from build123d import *

# Parameters (mm, degrees)
F0_W      = 146.05
F0_H      = 127
F1_DEPTH  = 2.54
F2_W      = 146.05
F2_H      = 12.7
F3_DEPTH  = 50.8
F5_W      = 50.8
F5_H      = 28.575
F6_DEPTH  = 12.7
F7_W      = 50.8
F7_H      = 3.175
F7_H_2    = 12.7
F8_DEPTH  = 1.5875
F9_W      = 63.5
F9_H      = 50.8
F10_DEPTH = 2.54
F11_W     = 12.7
F11_H     = 73.025
F12_DEPTH = 50.8
F13_W     = 148.59
F13_H     = 2.54
F15_DEPTH = 57.15
F14_W     = 2.54
F14_H     = 127
F16_DEPTH = 57.15
F18_DEPTH = 50.8
F19_W     = 31.75
F19_H     = 12.7
F20_DEPTH = 50.8
F22_DEPTH = 50.8
F24_DEPTH = 50.8
F25_W     = 12.68959
F25_H     = 50.8
F26_DEPTH = 50.8
F4_W      = 15.875
F4_H      = 15.875
F27_DEPTH = 38.1
F28_W     = 85.09
F28_H     = 2.54
F29_DEPTH = 57.15
F30_W     = 2.54
F30_H     = 50.8
F32_DEPTH = 57.15
F31_W     = 63.5
F31_H     = 2.54
F33_DEPTH = 57.15
F34_W     = 2.54
F34_H     = 57.15
F35_DEPTH = 57.15


with BuildPart() as f1:
    # F0 (on Top) → F1 (new body)
    with BuildSketch(Plane.XY):
        Rectangle(F0_W, F0_H)
    extrude(amount=F1_DEPTH)

    # F2 (on face) → F3 (join)
    with BuildSketch(Plane.XY.offset(2.54)):
        with Locations((0, 57.15)):
            Rectangle(F2_W, F2_H)
    extrude(amount=F3_DEPTH)

    # F5 (on face) → F6 (cut)
    with BuildSketch(Plane.XZ.offset(-50.8)):
        with Locations((0, 35.8775)):
            Rectangle(F5_W, F5_H)
    extrude(amount=-F6_DEPTH, mode=Mode.SUBTRACT)

    # F7 (on face) → F8 (join)
    with BuildSketch(Plane.XY.offset(21.59)):
        with Locations((0, 49.2125)):
            Rectangle(F7_W, F7_H)
        with Locations((0, 57.15)):
            Rectangle(F7_W, F7_H_2)
    extrude(amount=F8_DEPTH)

    # F9 (on Top) → F10 (join)
    with BuildSketch(Plane.XY):
        with Locations((-41.275, -88.9)):
            Rectangle(F9_W, F9_H)
    extrude(amount=F10_DEPTH)

    # F11 (on face) → F12 (join)
    with BuildSketch(Plane.XY.offset(2.54)):
        with Locations((66.675, 14.2875)):
            Rectangle(F11_W, F11_H)
    extrude(amount=F12_DEPTH)

    # F13 (on Top) → F15 (join)
    with BuildSketch(Plane.XY):
        with Locations((1.27, 64.77)):
            Rectangle(F13_W, F13_H)
    extrude(amount=F15_DEPTH)

    # F14 (on Top) → F16 (join)
    with BuildSketch(Plane.XY):
        with Locations((74.295, 0)):
            Rectangle(F14_W, F14_H)
    extrude(amount=F16_DEPTH)

    # F17 (on face) → F18 (join)
    with BuildSketch(Plane.XY.offset(2.54)):
        Polygon((60.325, 31.75), (60.325, 50.8), (41.275, 50.8), align=None)
    extrude(amount=F18_DEPTH)

    # F19 (on face) → F20 (join)
    with BuildSketch(Plane.XY.offset(2.54)):
        with Locations((6.35, -57.15)):
            Rectangle(F19_W, F19_H)
    extrude(amount=F20_DEPTH)

    # F21 (on face) → F22 (join)
    with BuildSketch(Plane.XY.offset(2.54)):
        Polygon((34.925, -63.5), (22.225, -50.8), (22.225, -63.5), align=None)
    extrude(amount=F22_DEPTH)

    # F23 (on face) → F24 (join)
    with BuildSketch(Plane.XY.offset(2.54)):
        Polygon((-9.525, -63.5), (-9.525, -50.8), (-22.21459, -63.5), align=None)
    extrude(amount=F24_DEPTH)

    # F25 (on face) → F26 (join)
    with BuildSketch(Plane.XY.offset(2.54)):
        with Locations((-15.869795, -88.9)):
            Rectangle(F25_W, F25_H)
    extrude(amount=F26_DEPTH)

    # F4 (on face) → F27 (join)
    with BuildSketch(Plane.XY.offset(2.54)):
        with Locations((65.0875, -36.5125)):
            Rectangle(F4_W, F4_H)
    extrude(amount=F27_DEPTH)

    # F28 (on Top) → F29 (join)
    with BuildSketch(Plane.XY):
        with Locations((33.02, -64.77)):
            Rectangle(F28_W, F28_H)
    extrude(amount=F29_DEPTH)

    # F30 (on Top) → F32 (join)
    with BuildSketch(Plane.XY):
        with Locations((-8.255, -91.44)):
            Rectangle(F30_W, F30_H)
    extrude(amount=F32_DEPTH)

    # F31 (on Top) → F33 (join)
    with BuildSketch(Plane.XY):
        with Locations((-41.275, -115.57)):
            Rectangle(F31_W, F31_H)
    extrude(amount=F33_DEPTH)

    # F34 (on Top) → F35 (join)
    with BuildSketch(Plane.XY):
        with Locations((-74.295, -88.265)):
            Rectangle(F34_W, F34_H)
    extrude(amount=F35_DEPTH)


solid = f1.part
Geometry: final body of the model. Coordinates: model frame, mm. A direction names the side the tool comes from. Round coordinates to 2 decimals unless told otherwise and drop trailing zeros. Loops run counter-clockwise (first coordinate to the right, second up) from the corner with the lowest first, then second, coordinate; pieces in that order, holes last.
Q1. Access query for faces 1 (the flat face through (-1, 63.5, 55)), 2 (the flat face through (25.4, 57, 36)), 3 (the flat face through (-22.215, -89, 28)), 4 (the flat face through (-73.025, 54, 20)). Directions: +Z, -Z, +X, -X, +Y, -Y. A direction counts if a zero-diameter tool reaches every point of the face in a straight line with its end or side. Return the directions, or none.
Q2. Section D-D on x = 38. Return loops of the section in (y, z).
Q3. Pull-direction query (Y, two-part tool) for faces 5 (the flat face through (-6.985, -92, 28)), 6 (the flat face through (0, 66.04, 28)), 7 (the flat face through (65, -44.45, 21)), 8 (the flat face through (67, -22.225, 28)); classes: released by +Y, released by -Y, zero draft, split by the parting line, or undercut.
Q4. Material intervals for L1, parallel to Y at x = 61, z = 18 (3 decimals); L2, parallel to Y at x = 40.5, z = 9.5; L3, parallel to Y at x = -33, z = 35.5, sorted ascending.
Q5. Pin query (flat end, axial travel): P1, Ø4, axis at x = 67.5, z = 39.5, coming from the -Y side; P2, Ø5, axis at x = -3.5, y = 55, coming from the +Z side; P3, Ø8, axis at y = -36, z = 24, coming from the -X side. Return the tip coordinate at first contact, or that it passes through.
Q6. Section C-C on y = 25. Return loops of the section in (x, z) (3 decimals).
Q7. Section B-B on z = 28. Return loops of the section in (x, y) (3 decimals), plus the area to 3 significant figures.
Evaluation:
1. face 1: +Z, -X
1. face 2: none
1. face 3: +Z
1. face 4: +Z, -Z, -X, +Y
2. outline: (-66.04, 0) - (66.04, 0) - (66.04, 57.15) - (63.5, 57.15) - (63.5, 53.34) - (50.8, 53.34) - (50.8, 2.54) - (-63.5, 2.54) - (-63.5, 57.15) - (-66.04, 57.15) - close
3. face 5: zero draft
3. face 6: released by +Y
3. face 7: undercut
3. face 8: undercut
4. L1: y = -66.04 to -63.5, -44.45 to -28.575, -22.225 to 66.04
4. L2: y = -66.04 to -63.5, 50.8 to 66.04
4. L3: y = -116.84 to -114.3, 50.8 to 66.04
5. P1: stops at y = -66.04
5. P2: stops at z = 53.34
5. P3: stops at x = 57.15
6. outline: (-73.025, 0) - (75.565, 0) - (75.565, 57.15) - (73.025, 57.15) - (73.025, 53.34) - (60.325, 53.34) - (60.325, 2.54) - (-73.025, 2.54) - close
7. outline: (-75.565, -116.84) - (-6.985, -116.84) - (-6.985, -66.04) - (75.565, -66.04) - (75.565, 66.04) - (-73.025, 66.04) - (-73.025, 50.8) - (-25.4, 50.8) - (-25.4, 63.5) - (25.4, 63.5) - (25.4, 50.8) - (41.275, 50.8) - (60.325, 31.75) - (60.325, -22.225) - (73.025, -22.225) - (73.025, -28.575) - (57.15, -28.575) - (57.15, -44.45) - (73.025, -44.45) - (73.025, -63.5) - (34.925, -63.5) - (22.225, -50.8) - (-9.525, -50.8) - (-22.215, -63.5) - (-22.215, -114.3) - (-73.025, -114.3) - (-73.025, -59.69) - (-75.565, -59.69) - close
7. area: 5,130 mm2
